Geometry: final body of the model. Coordinates: model frame, mm. A direction names the side the tool comes from. Round coordinates to 2 decimals unless told otherwise and drop trailing zeros. Order: outer loops, then holes, each group sorted by start corner. A loop starts at its lowest first (then second) coordinate and runs counter-clockwise, first axis right, second up. Notation, with made-up numbers: M 88,-6 L 133,-6 A21 cw 133,14 Z; hole C 86.5,-9 d1. An arc over 180 degrees is marked long. Put each result on its own line as item: value. Start each with the question number.
1) Section D-D, the plane z = 23.5. Return loops of the section in (x, y), then the cut area to 3 significant figures.
2) Section B-B, the plane x = 44.5. Return loops of the section in (y, z), then the cut area to 3 significant figures.
3) Material intervals for probe 1 along Z at (x, y) = (34, 46); probe 2 along X at (y, z) = (-2, 43.5); probe 3 along Z at (x, y) = (25, 23), sorted ascending. Write a range as [from, to].
4) Section A-A, the plane y = -27. Return loops of the section in (x, z), then the cut area to 3 significant figures.
5) Draft query along Y for faces 1 (the flat face through (0, -1, 26)), 2 (the flat face through (34, 54, -50)), 3 (the cylindrical face through (7.4, -37.74, 27.93)). Return one class per face: pulls with the +Y half, pulls with the -Y half, needs draft (parallel to the pull), parting line crosses it, or undercut.
6) First-contact query: P1, Ø4, axis at x = 34.5, y = 5, coming from the +Z side; P2, Ø8, axis at y = -40.5, z = 41.5, coming from the +X side; P3, Ø1, axis at x = 46, z = -51, coming from the -Y side; P4, Ø12, axis at y = -3, z = 48, coming from the -X side. Flat tips, straight axial feed; report the tip coordinate or a pass-through.
7) Section C-C, the plane z = 51.5. Return loops of the section in (x, y), then the cut area to 3 significant figures.
8) Access query for faces 4 (the flat face through (39, 27, 0)), 5 (the flat face through (58, -37, 2)), 6 (the flat face through (34, 44, -45)), 7 (the flat face through (30, -27, 5)). Directions: +Z, -Z, +X, -X, +Y, -Y. A direction counts if a zero-diameter tool reaches every point of the face in a straight line with its end or side. Return the directions, or none.
from build123d import *

# Parameters (mm, degrees)
BOSS_EXTRUDE1_DEPTH = 10
SKETCH2_3_W         = 54
SKETCH2_3_H         = 54
SKETCH2_3_R         = 11
BOSS_EXTRUDE2_DEPTH = 15
SKETCH3_W           = 15
SKETCH3_H           = 108
BOSS_EXTRUDE3_DEPTH = 10
BOSS_EXTRUDE4_DEPTH = 54
SKETCH5_W           = 54
SKETCH5_H           = 54
BOSS_EXTRUDE5_DEPTH = 5
SKETCH8_W           = 69
SKETCH8_H           = 10
BOSS_EXTRUDE6_DEPTH = 54
SKETCH10_R          = 34.395117581
SKETCH10_R_2        = 13.5
BOSS_EXTRUDE7_DEPTH = 10
SKETCH11_R          = 13.5
CUT_EXTRUDE1_DEPTH  = 10
SKETCH12_W          = 38
SKETCH12_H          = 20
CUT_EXTRUDE2_DEPTH  = 12
BOSS_EXTRUDE9_DEPTH = 20


with BuildPart() as part:
    # Sketch2 → Boss-Extrude1 (new body)
    with BuildSketch(Plane(origin=(0, 0, 0), x_dir=(0, 0, -1), z_dir=(1, 0, 0))):
        Polygon((0, 54), (-54, 0), (0, 0), align=None)
    extrude(amount=BOSS_EXTRUDE1_DEPTH)

    # Sketch2_3 → Boss-Extrude2 (add)
    # profile 1 of 2: a face of its own
    with BuildSketch(Plane(origin=(0, 0, 0), x_dir=(0, 0, -1), z_dir=(1, 0, 0))):
        with Locations((-27, -27)):
            Rectangle(SKETCH2_3_W, SKETCH2_3_H)
        with Locations((-25.545100882, -27)):
            Circle(SKETCH2_3_R, mode=Mode.SUBTRACT)
    # profile 2 of 2: a face of its own
    with BuildSketch(Plane(origin=(0, 0, 0), x_dir=(0, 0, -1), z_dir=(1, 0, 0))):
        with BuildLine():
            Line((-54, 0), (-54, -54))
            ThreePointArc((-54, -54), (-81, -27), (-54, 0))
        make_face()
    extrude(amount=BOSS_EXTRUDE2_DEPTH)

    # Sketch3 → Boss-Extrude3 (add)
    with BuildSketch(Plane(origin=(0, 0, 0), x_dir=(-1, 0, 0), z_dir=(0, 0, -1))):
        with Locations((-7.5, 0)):
            Rectangle(SKETCH3_W, SKETCH3_H)
    extrude(amount=BOSS_EXTRUDE3_DEPTH)

    # Sketch4 → Boss-Extrude4 (add)
    with BuildSketch(Plane(origin=(15, 0, 0), x_dir=(0, 0, -1), z_dir=(1, 0, 0))):
        Polygon((10, 54), (0, 54), (0, 0), (0, -54), (10, -54), align=None)
    extrude(amount=BOSS_EXTRUDE4_DEPTH)

    # Sketch5 → Boss-Extrude5 (add)
    with BuildSketch(Plane.XY):
        with Locations((42, -27)):
            Rectangle(SKETCH5_W, SKETCH5_H)
    extrude(amount=BOSS_EXTRUDE5_DEPTH)

    # Sketch8 → Boss-Extrude6 (add)
    with BuildSketch(Plane(origin=(0, 0, -10), x_dir=(-1, 0, 0), z_dir=(0, 0, -1))):
        with Locations((-34.5, 49)):
            Rectangle(SKETCH8_W, SKETCH8_H)
    extrude(amount=BOSS_EXTRUDE6_DEPTH)

    # Sketch10 → Boss-Extrude7 (add)
    with BuildSketch(Plane(origin=(0, 54, 0), x_dir=(1, 0, 0), z_dir=(0, 1, 0))):
        with Locations((34.5, 64)):
            Circle(SKETCH10_R)
        with Locations((34.5, 64)):
            Circle(SKETCH10_R_2, mode=Mode.SUBTRACT)
    extrude(amount=-BOSS_EXTRUDE7_DEPTH)

    # Sketch11 → Cut-Extrude1 (cut)
    with BuildSketch(Plane(origin=(0, 54, 0), x_dir=(1, 0, 0), z_dir=(0, 1, 0))):
        with Locations(Location((34.5, 64, 0), (0, 0, 270))):
            Circle(SKETCH11_R)
    extrude(amount=-CUT_EXTRUDE1_DEPTH, mode=Mode.SUBTRACT)

    # Sketch12 → Cut-Extrude2 (cut)
    with BuildSketch(Plane.XY.offset(5)):
        with Locations((50, -27)):
            Rectangle(SKETCH12_W, SKETCH12_H)
    extrude(amount=-CUT_EXTRUDE2_DEPTH, mode=Mode.SUBTRACT)

    # Sketch14 → Boss-Extrude9 (add)
    with BuildSketch(Plane(origin=(0, -37, 0), x_dir=(1, 0, 0), z_dir=(0, 1, 0))):
        Polygon((31, -5), (69, 7), (31, 7), align=None)
    extrude(amount=BOSS_EXTRUDE9_DEPTH)


solid = part.part
Result sheet:
1. outline: M 0,-54 L 15,-54 L 15,-37.81 L 0,-37.81 Z; M 0,-16.19 L 15,-16.19 L 15,0 L 10,0 L 10,30.5 L 0,30.5 Z
1. area: 791 mm2
2. outline: M -54,-10 L 44,-10 L 44,-54.93 L 54,-54.93 L 54,0 L 0,0 L 0,5 L -17,5 L -17,0.74 L -37,0.74 L -37,5 L -54,5 Z; M 44,-96.91 L 54,-96.91 L 54,-73.07 L 44,-73.07 Z
2. area: 1,950 mm2
3. probe 1: z = [-98.39, -77.49], [-50.51, 0]
3. probe 2: x = [0, 15]
3. probe 3: z = [-10, 0]
4. outline: M 0,-10 L 69,-10 L 69,-7 L 31,5 L 15,5 L 15,14.55 L 0,14.55 Z; M 0,36.55 L 15,36.55 L 15,81 L 0,81 Z
4. area: 1,620 mm2
5. face 1: needs draft
5. face 2: pulls with the +Y half
5. face 3: undercut
6. P1: stops at z = 0
6. P2: stops at x = 15
6. P3: stops at y = 44
6. P4: stops at x = 0
7. outline: M 0,-54 L 15,-54 L 15,0 L 10,0 L 10,2.5 L 0,2.5 Z
7. area: 835 mm2
8. face 4: +Z, +X, +Y
8. face 5: +Z, +X
8. face 6: -Z, +X, -X, -Y
8. face 7: +Z, +X, +Y, -Y
